Input: part model. Units: mm. Frame: model coordinates. A direction names the side the tool comes from. Give positions to 0.01 mm unless a question says otherwise; leave off trailing zeros. Loops run counter-clockwise (first coordinate to the right, second up) from the corner with the lowest first, then second, coordinate; pieces in that order, holes last. Notation, with made-up numbers: M -13,-21 L 6,-21 A3 ccw 6,-16 Z; hole C 71,46 d9. An arc over 180 degrees is marked long. Answer as a JSON object with one key per item and string values. Group by question number.
1) Ray query, L1, parallel to Z at x = 12.5, y = 30.25; L2, parallel to X at y = 33, z = 0; L3, parallel to Y at x = -1.5, z = 6.5. Return the intervals inside material, ascending.
2) Section query C-C on y = 37. Return loops of the section in (x, z), plus the area to 3 significant figures.
3) Access query for faces 4 (the flat face through (13.5, 39.4, 16)), 5 (the cylindrical face through (9.667, 2.218, -1.269)), 6 (the cylindrical face through (3.27, 63.83, 10.4)), 7 (the flat face through (-14, 50, -11.5)). Directions: +Z, -Z, +X, -X, +Y, -Y. A direction counts if a zero-diameter tool reaches every point of the face in a straight line with its end or side. Return the directions, or none.
4) Draft query along Z for faces 1 (the cylindrical face through (-15.62, 31.85, -18.22)), 2 (the cylindrical face through (11.579, 31.846, 15.845)), 3 (the flat face through (-13, 39.4, -17)). Return one class per face: +Z half, -Z half, draft (parallel to the pull), parting line (faces both ways), or undercut.
5) First-contact query: P1, Ø4, axis at y = 15.5, z = 6, coming from the -X side; P2, Ø1.9, axis at y = 45.5, z = 16.5, coming from the +X side; P3, Ø1.1, axis at y = 52, z = -16.5, coming from the -X side. Flat tips, straight axial feed; report the tip coordinate or a pass-through.
6) Section query D-D on y = 5.5. Return loops of the section in (x, z), plus the area to 3 significant figures.
from build123d import *

# Parameters (mm, degrees)
F2_W     = 79.127467
F2_H     = 78.408126
F2_W_2   = 32.5
F2_H_2   = 37.5
F3_DEPTH = 66.201
F5_DEPTH = 26.8
F7_D     = 2.5
F7_DEPTH = 50
F8_SIZE  = 1


with BuildPart() as f1:
    # F0 (on Right) → F1 (revolve)
    with BuildSketch(Plane.YZ):
        Polygon((24.5, 11), (4.5, 11), (4.5, 9.75), (0, 9.75), (0, 8), (15, 8), (15, 6), (50, 6), (50, 4), (66.2, 4), (66.2, 10.9), (62.5, 10.9), (62.5, 12.5), (55.031813, 24), (24.5, 24), align=None)
    revolve(axis=Axis((0, 44.76735, 0), (0, 1, 0)))

    # F2 (on face) → F3 (cut, through all)
    with BuildSketch(Plane(origin=(0, 66.2, 0), x_dir=(-1, 0, 0), z_dir=(0, 1, 0))):
        with Locations((1.602461, -2.474608)):
            Rectangle(F2_W, F2_H)
        Rectangle(F2_W_2, F2_H_2, mode=Mode.SUBTRACT)
    extrude(amount=-F3_DEPTH, mode=Mode.SUBTRACT)

    # F4 (on face) → F5 (cut)
    with BuildSketch(Plane(origin=(0, 66.2, 0), x_dir=(-1, 0, 0), z_dir=(0, 1, 0))):
        with BuildLine():
            Line((-18, 11.501228), (-12.592719, 11.501228))
            ThreePointArc((-12.592719, 11.501228), (-10.058127, 12.492559), (-9, 15))
            Line((-9, 15), (-9, 21))
            Line((-9, 21), (-18, 21))
            Line((-18, 21), (-18, 11.501228))
        make_face()
        with BuildLine():
            Line((18, -11.5), (12.5, -11.5))
            ThreePointArc((12.5, -11.5), (10.025126, -12.525126), (9, -15))
            Line((9, -15), (9, -21))
            Line((9, -21), (18, -21))
            Line((18, -21), (18, -11.5))
        make_face()
    extrude(amount=-F5_DEPTH, mode=Mode.SUBTRACT)

    # F7
    with Locations(Plane(origin=(0, 39.4, 0), x_dir=(-1, 0, 0), z_dir=(0, 1, 0))):
        with Locations((-12.5, 15), (12.5, -15)):
            Hole(F7_D / 2, depth=F7_DEPTH)

    # F8
    f8_edges = [f1.edges().sort_by_distance(p)[0] for p in [
        (0, 66.2, -10.9),
    ]]
    chamfer(f8_edges, length=F8_SIZE)


solid = f1.part
Output:
{
 "1": {"L1": "z = -18.75 to 13.75, 16.25 to 18.75", "L2": "x = -16.25 to -6, 6 to 16.25", "L3": "y = 15 to 66.2"},
 "2": {"outline": "M -16.25,-17.66 A24 ccw -14.98,-18.75 L 14.98,-18.75 A24 ccw 16.25,-17.66 L 16.25,17.66 A24 ccw 14.98,18.75 L -14.98,18.75 A24 ccw -16.25,17.66 Z; hole C -12.5,-15 d2.5; hole C 0,0 d12; hole C 12.5,15 d2.5", "area": "1,090 mm^2"},
 "3": {"face 4": "+Z, +X, +Y", "face 5": "-Y", "face 6": "+Y", "face 7": "-Z, -X, +Y"},
 "4": {"face 1": "-Z half", "face 2": "undercut", "face 3": "draft"},
 "5": {"P1": "stops at x = -10.25", "P2": "stops at x = 9", "P3": "stops at x = -9"},
 "6": {"outline": "C 0,0 d22; hole C 0,0 d16", "area": "179 mm^2"}
}
